Work out the finished part from the listing and answer in its coordinate system (mm). A direction names the side the tool comes from. Give positions to 0.01 mm unless a question says otherwise; leave off trailing zeros. Write each loop counter-clockwise with the first axis right and the second up, starting at its lowest first coordinate (ties: lowest second). Pieces come first, ordered by that corner, then holes.
1) A tool of negligible diameter and unlimited length cuts with its end or side. For faces 1 (the face through (3, 8.742, 2)), 2 (the face through (-40, -14.058, 2)), 3 (the face through (-8.37, -22.34, 1.48)), from which of +Z, -Z, +X, -X, +Y, -Y can it reach the whole face along a straight path? Write none if from no direction.
2) Find section D-D (y = 3.5). Determine the outline of the cut face in (x, z), plus the area to 3 significant figures.
3) Find section C-C (y = -48). Determine the outline of the cut face in (x, z), plus the area to 3 significant figures.
4) Find section B-B (z = 2.05). Count the separate pieces of the cut face and the enclosed holes in it, plus the area to 3 significant figures.
5) Straight lines are drawn through the part: probe 1 along X at (y, z) = (6, 0.8); probe 2 along Y at (x, z) = (-7, 0.75); probe 3 along Y at (x, z) = (-22, 2.15). For each, find the intervals that lie inside material, in ascending order.
6) Given pin 1 Ø3 at (x, y) = (-25.49, -20.66) entering from +Z; pin 2 Ø1.5 at (y, z) = (-22, 1.5) entering from -X; pin 3 Ø0.9 at (y, z) = (-2.5, 1) entering from +X, each flat-ended and moving along its own axis, determine where each tip first touches the part or whether it passes through.
7) Find section A-A (x = -7). Determine the outline of the cut face in (y, z).
8) Determine the mould class of faces 4 (the face through (-18, 16.542, 1)), 5 (the face through (-40.993, -10, 1)), 6 (the face through (-40, -29.058, 2)) for opening direction Y: pulls with the +Y half, pulls with the -Y half, needs draft (parallel to the pull), parting line crosses it, or undercut.
```python
from build123d import *

# Parameters (mm, degrees)
SKETCH1_W             = 46
SKETCH1_H             = 76.2
BOSS_EXTRUDE1_DEPTH   = 3
SKETCH2_W             = 3
SKETCH2_H             = 15
CUT_EXTRUDE1_DEPTH    = 73.446802019
LPATTERN1_COUNT       = 3
LPATTERN1_PITCH       = 22.8
F_6_CLEARANCE_HOLE1_D = 3.7973
CUT_EXTRUDE2_REACH    = 74.447
SKETCH5_R             = 5


with BuildPart() as part:
    # Sketch1 → Boss-Extrude1 (new body)
    with BuildSketch(Plane.XY):
        with Locations((-17.993460648, -21.557986111)):
            Rectangle(SKETCH1_W, SKETCH1_H)
    extrude(amount=BOSS_EXTRUDE1_DEPTH)

    # Sketch2 → Cut-Extrude1 (cut, through all)
    with BuildSketch(Plane.XY.offset(3)):
        with Locations((-39.493460648, 1.242013889)):
            Rectangle(SKETCH2_W, SKETCH2_H)
        with Locations((3.506539352, 1.242013889)):
            Rectangle(SKETCH2_W, SKETCH2_H)
    cut_extrude1 = extrude(amount=-CUT_EXTRUDE1_DEPTH, mode=Mode.SUBTRACT)

    # LPattern1: Cut-Extrude1 ×3
    with Locations(*[(0, -i * LPATTERN1_PITCH, 0) for i in range(1, LPATTERN1_COUNT)]):
        add(cut_extrude1, mode=Mode.SUBTRACT)

    # #6 Clearance Hole1 (through all)
    with Locations(Plane.XY.offset(3)):
        with Locations((-25.493460648, -20.657986111), (-7.493460648, -20.657986111)):
            Hole(F_6_CLEARANCE_HOLE1_D / 2)

    # Sketch5 → Cut-Extrude2 (cut, up to next)
    with BuildSketch(Plane(origin=(0, 0, 0), x_dir=(-1, 0, 0), z_dir=(0, 0, -1)), mode=Mode.PRIVATE) as cut_extrude2_sk1:
        with Locations((17.993460648, -44.357986111)):
            Circle(SKETCH5_R)
    cut_extrude2_tool1 = extrude(cut_extrude2_sk1.sketch, amount=-CUT_EXTRUDE2_REACH, mode=Mode.PRIVATE) & part.part
    add(cut_extrude2_tool1.solids().sort_by_distance((-17.993461, -44.357986, 0))[0], mode=Mode.SUBTRACT)


solid = part.part
```
Results:
1. face 1: +Z, -Z, +X
1. face 2: +Z, -Z, -X
1. face 3: +Z, -Z
2. outline: (-37.99, 0) - (2.01, 0) - (2.01, 3) - (-37.99, 3) - close
2. area: 120 mm2
3. outline: (-37.99, 0) - (-21.42, 0) - (-21.42, 3) - (-37.99, 3) - close; (-14.57, 0) - (2.01, 0) - (2.01, 3) - (-14.57, 3) - close
3. area: 99.4 mm2
4. separate pieces: 1
4. enclosed holes: 3
4. area: 3,130 mm2
5. probe 1: x = -37.99 to 2.01
5. probe 2: y = -59.66 to -22.49, -18.82 to 16.54
5. probe 3: y = -59.66 to -47.35, -41.37 to 16.54
6. pin 1: passes through
6. pin 2: stops at x = -37.99
6. pin 3: stops at x = 2.01
7. outline: (-59.66, 0) - (-22.49, 0) - (-22.49, 3) - (-59.66, 3) - close; (-18.82, 0) - (16.54, 0) - (16.54, 3) - (-18.82, 3) - close
8. face 4: pulls with the +Y half
8. face 5: needs draft
8. face 6: undercut
